Design review of the part built by this model. Coordinates are the model's own, in mm. Face numbers are marked on the shaded views. A direction names the side the tool comes from. Give positions to 0.01 mm unless a question says otherwise; leave off trailing zeros. Order: outer loops, then holes, each group sorted by start corner. A loop starts at its lowest first (then second) coordinate and runs counter-clockwise, first axis right, second up. Notation, with made-up numbers: (55, 86.25) -> (59, 86.25) arc R17 cw to (59, 107.25) -> close; hole circle Ø6 at (2.5, 85). An arc over 180 degrees is marked (long way). One line per item, written item: value. Start each with the question number.
1) Consider section D-D (z = 1.75). State the section outline as (x, y) points.
2) Tool access review of the marked faces 1, 2, 3, 4 and 5: name each direction out of +Z, -Z, +X, -X, +Y, -Y from which nothing blocks a thin tool from reaching the whole face with its end or side.
3) Consider section C-C (y = 3.75). State the section outline as (x, z) points.
4) Consider section B-B (x = 7.25). State the section outline as (y, z) points.
5) Consider section A-A (y = -4). State the section outline as (x, z) points.
6) The part is to be moulded in two halves that separate along X. For the marked faces 6, 7 and 8, say which applies: released by +X, released by -X, zero draft, split by the parting line, or undercut.
7) For pin 1 (2 mm diameter, centred on y = 2, z = 0, fed in from -X); pin 2 (1 mm diameter, centred on x = 6.5, z = -3, fed in from -Y); pin 3 (4 mm diameter, centred on y = -3.5, z = -1, fed in from +X), all flat-tipped, find the tip position at first contact; note any pin that passes through.
8) Wall thickness on line 1 along X through (y, z) = (-1.5, -3); line 2 along Y through (x, z) = (15, 1); line 3 along X through (y, z) = (-1, -0.25): over which ranges is each line inside the solid? List them lowest first. Write a range as from..to.
from build123d import *

# Parameters (mm, degrees)
SKETCH_1_W               = 22
SKETCH_1_H               = 5
CUT_EXTRUDE_1_DEPTH      = 24.108440017
CUT_EXTRUDE_1_DEPTH_BACK = 24.108440017
SKETCH_3_W               = 4
SKETCH_3_H               = 5
CUT_EXTRUDE_4_DEPTH      = 24.108440017
CUT_EXTRUDE_4_DEPTH_BACK = 24.108440017
SKETCH_4_W               = 14
SKETCH_4_H               = 5
CUT_EXTRUDE_5_DEPTH      = 24.108440017
CUT_EXTRUDE_5_DEPTH_BACK = 16
SKETCH_5_R               = 2
SKETCH_6_W               = 10.5
SKETCH_6_H               = 3.627911102
CUT_EXTRUDE_6_DEPTH      = 16


with BuildPart() as part:
    # 草图1 → 旋转1 (revolve)
    with BuildSketch(Plane.XY):
        with Locations((11, 2.5)):
            Rectangle(SKETCH_1_W, SKETCH_1_H)
    revolve(axis=Axis((22, 0, 0), (-1, 0, 0)))

    # 草图3 → 切除-拉伸1 (cut, two sides: drawn at the far end of the back side and taken through both)
    with BuildSketch(Plane.XY.offset(-CUT_EXTRUDE_1_DEPTH_BACK)):
        with Locations((20, -2.5)):
            Rectangle(SKETCH_3_W, SKETCH_3_H)
        Polygon((22, 0.5), (18, 5), (22, 5), align=None)
    extrude(amount=CUT_EXTRUDE_1_DEPTH + CUT_EXTRUDE_1_DEPTH_BACK, mode=Mode.SUBTRACT)

    # 草图4 → 切除-拉伸4 (cut, two sides: drawn at the far end of the back side and taken through both)
    with BuildSketch(Plane(origin=(0, 0, 0), x_dir=(1, 0, 0), z_dir=(0, 1, 0)).offset(-CUT_EXTRUDE_4_DEPTH_BACK)):
        with Locations((7, -2.5)):
            Rectangle(SKETCH_4_W, SKETCH_4_H)
    extrude(amount=CUT_EXTRUDE_4_DEPTH + CUT_EXTRUDE_4_DEPTH_BACK, mode=Mode.SUBTRACT)

    # 草图5 → 切除-拉伸5 (cut, two sides: drawn at the far end of the back side and taken through both)
    with BuildSketch(Plane.ZY.offset(-CUT_EXTRUDE_5_DEPTH_BACK)):
        with Locations(Location((0, 2, 0), (0, 0, 270))):
            Circle(SKETCH_5_R)
    extrude(amount=CUT_EXTRUDE_5_DEPTH + CUT_EXTRUDE_5_DEPTH_BACK, mode=Mode.SUBTRACT)

    # 草图6 → 切除-拉伸6 (cut)
    with BuildSketch(Plane.XY):
        with Locations((6.75, -3.186044449)):
            Rectangle(SKETCH_6_W, SKETCH_6_H)
    extrude(amount=-CUT_EXTRUDE_6_DEPTH, mode=Mode.SUBTRACT)


solid = part.part
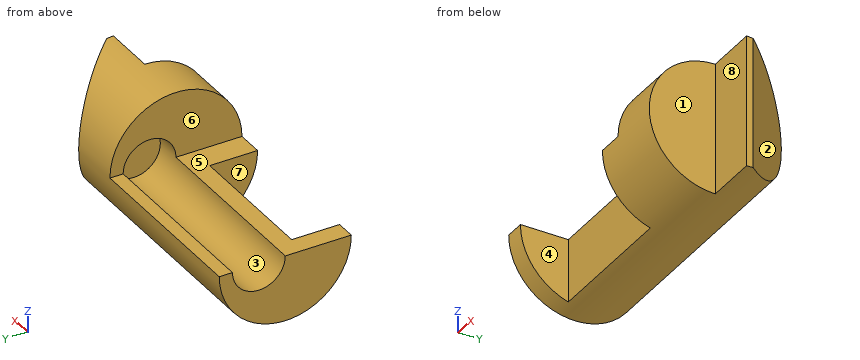
Checked values:
1. outline: (14, -4.68) -> (18, -4.68) -> (18, 0) -> (22, 0) -> (22, 0.5) -> (18.28, 4.68) -> (14, 4.68) -> (14, 2.97) -> (16, 2.97) -> (16, 1.03) -> (14, 1.03) -> close
2. face 1: +Z, -Z, +X, -Y
2. face 2: +Z, -Z, +X, +Y
2. face 3: -X
2. face 4: +Z, -Z, -Y
2. face 5: +Z, -X, +Y, -Y
3. outline: (0, -3.31) -> (19.11, -3.31) -> (19.11, 3.31) -> (14, 3.31) -> (14, 0.97) -> (16, 0.97) -> (16, -0.97) -> (0, -0.97) -> close
4. outline: (-1.37, -4.81) arc R5 ccw to (5, 0) -> (4, 0) arc R2 cw to (0, 0) -> (-1.37, 0) -> close
5. outline: (0, -3) -> (1.5, -3) -> (1.5, 0) -> (0, 0) -> close; (12, -3) -> (18, -3) -> (18, 3) -> (14, 3) -> (14, 0) -> (12, 0) -> close
6. face 6: released by -X
6. face 7: undercut
6. face 8: zero draft
7. pin 1: stops at x = 16
7. pin 2: stops at y = -1.37
7. pin 3: stops at x = 18
8. line 1: x = 0..1.5, 12..18
8. line 2: y = -4.9..0.27, 3.73..4.9
8. line 3: x = 0..18
